from build123d import *

# Parameters (mm, degrees)
SKETCH1_R           = 43.4
BOSS_EXTRUDE1_DEPTH = 13.3
SKETCH3_R           = 1.5
SKETCH3_R_2         = 2
CUT_EXTRUDE1_DEPTH  = 10
SKETCH4_R           = 1.5
CUT_EXTRUDE2_DEPTH  = 5


with BuildPart() as part:
    # Sketch1 → Boss-Extrude1 (new, symmetric)
    with BuildSketch(Plane.XY):
        Circle(SKETCH1_R)
    extrude(amount=BOSS_EXTRUDE1_DEPTH, both=True)

    # Sketch2 → Cut-Revolve1 (revolve, cut)
    with BuildSketch(Plane(origin=(0, 0, 0), x_dir=(1, 0, 0), z_dir=(0, 1, 0))):
        Polygon((-43.4, -7.3), (-22.5, -13.3), (-43.4, -13.3), align=None)
        Polygon((-43.4, 9.3), (-43.4, 13.3), (-20, 13.3), (-40.4, 10.8), (-40.4, 9.3), align=None)
    revolve(axis=Axis((0, 0, -13.3), (0, 0, 1)), mode=Mode.SUBTRACT)

    # Sketch3 → Cut-Extrude1 (cut)
    with BuildSketch(Plane(origin=(0, 0, -13.3), x_dir=(-1, 0, 0), z_dir=(0, 0, -1))):
        with Locations((10.606601718, 10.606601718)):
            Circle(SKETCH3_R)
        with Locations((10.606601718, -10.606601718)):
            Circle(SKETCH3_R)
        with Locations((-10.606601718, -10.606601718)):
            Circle(SKETCH3_R)
        with Locations((-10.606601718, 10.606601718)):
            Circle(SKETCH3_R)
        with Locations((0, 16)):
            Circle(SKETCH3_R_2)
        with Locations((16, 0)):
            Circle(SKETCH3_R_2)
        with Locations((0, -16)):
            Circle(SKETCH3_R_2)
        with Locations((-16, 0)):
            Circle(SKETCH3_R_2)
    extrude(amount=-CUT_EXTRUDE1_DEPTH, mode=Mode.SUBTRACT)

    # Sketch4 → Cut-Extrude2 (cut)
    with BuildSketch(Plane.XY.offset(13.3)):
        with Locations((0, 17.5)):
            Circle(SKETCH4_R)
        with Locations((0, 12.5)):
            Circle(SKETCH4_R)
        with Locations((12.374368671, 12.374368671)):
            Circle(SKETCH4_R)
        with Locations((17.5, 0)):
            Circle(SKETCH4_R)
        with Locations((12.374368671, -12.374368671)):
            Circle(SKETCH4_R)
        with Locations((0, -17.5)):
            Circle(SKETCH4_R)
        with Locations((-12.374368671, -12.374368671)):
            Circle(SKETCH4_R)
        with Locations((-17.5, 0)):
            Circle(SKETCH4_R)
        with Locations((-12.374368671, 12.374368671)):
            Circle(SKETCH4_R)
        with Locations((12.5, 0)):
            Circle(SKETCH4_R)
        with Locations((0, -12.5)):
            Circle(SKETCH4_R)
        with Locations((-12.5, 0)):
            Circle(SKETCH4_R)
    extrude(amount=-CUT_EXTRUDE2_DEPTH, mode=Mode.SUBTRACT)


solid = part.part
Geometry: final body of the model. Coordinates: model frame, mm. A direction names the side the tool comes from. Coordinates: 2 decimals unless noted, no trailing zeros.
(1) Material intervals for probe 1 along Y at (x, z) = (16, -10.75); probe 2 along X at (y, z) = (-17, -10.75); probe 3 along X at (y, z) = (5.5, 4.75), sorted ascending.
(2) Access query for faces 4 (the face through (9.8, 11.87, -8.37)), 5 (the face through (0, 18, 8.3)). Directions: +Z, -Z, +X, -X, +Y, -Y. A direction counts if a zero-diameter tool reaches every point of the face in a straight line with its end or side. Return the directions, or none.
(3) Draft query along Y for faces 1 (the face through (-38.534, -12.135, -10.04)), 2 (the face through (0, 0, 13.3)), 3 (the face through (-12.7, 10.91, 10.84)). Return one class per face: pulls with the +Y half, pulls with the -Y half, needs draft (parallel to the pull), parting line crosses it, or undercut.
(4) First-contact query: pin 1 (5 mm diameter, centred on x = -2.5, z = 3.5, fed in from +Y); pin 2 (1.5 mm diameter, centred on x = -18, y = -0.5, fed in from +Z); pin 3 (1 mm diameter, centred on y = -24, z = -9.5, fed in from +X). Flat tips, straight axial feed; report the tip coordinate or a pass-through.
(5) Section query A-A (z = -5.25). State how many separate pieces and enclosed holes the cut face has, plus the area to 3 significant figures.
Solution:
1. probe 1: y = -37.1 to -2, 2 to 37.1
1. probe 2: x = -36.65 to -1.73, 1.73 to 36.65
1. probe 3: x = -43.05 to 43.05
2. face 4: -Z
2. face 5: +Z
3. face 1: parting line crosses it
3. face 2: needs draft
3. face 3: undercut
4. pin 1: stops at y = 43.4
4. pin 2: stops at z = 8.3
4. pin 3: stops at x = 36.46
5. separate pieces: 1
5. enclosed holes: 8
5. area: 5,840 mm2
